Study the drawing (mm; zero at the part's minimum x, y, z) and answer. A direction names the side the tool comes from. Round coordinates to 2 decimals unless told otherwise and drop trailing zeros. Write each loop counter-clockwise with the first axis right and the second up, starting at its lowest first coordinate (ties: lowest second). Pieces come first, ordered by that corner, then holes. Notation, with made-up numbers: M -27,45.25 L -13,45.25 A34 cw -13,79.25 Z; hole C 2,68 d7. An arc over 180 degrees is marked long. Put each result on its own line as item: value. Start each with the question number.
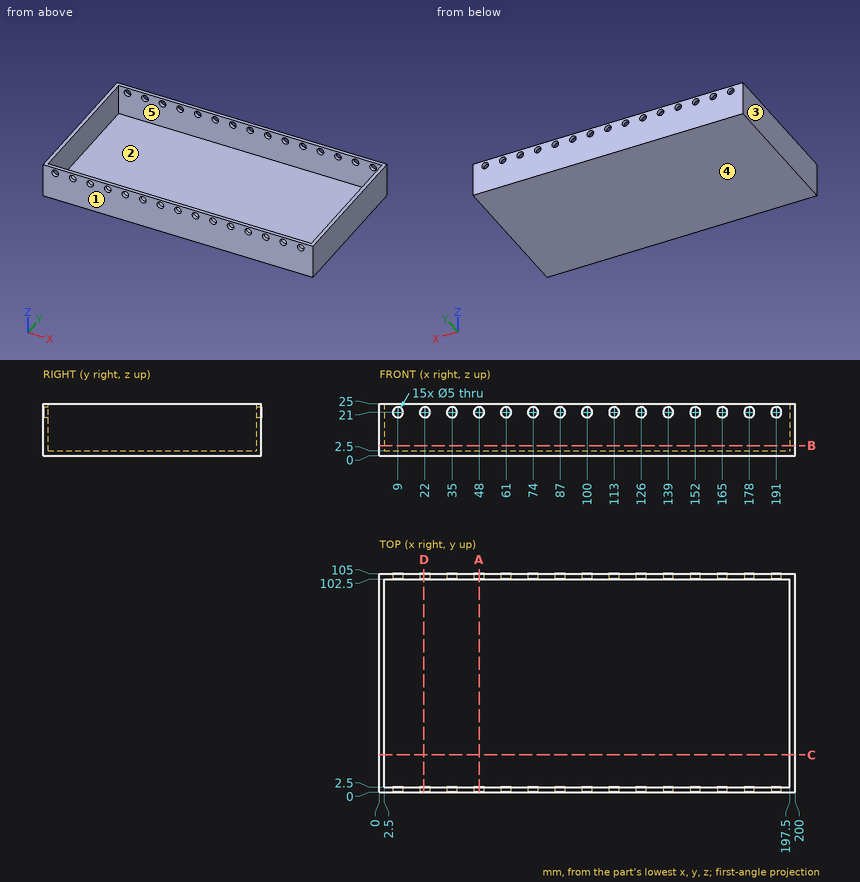
Item 1: Section A-A (x = 48) is taken. Give the vertices of the cut face in (y, z).
Item 2: Flat-ended cylindrical pins translate along their axes: pin 1 (3 mm diameter, centred on x = 176, y = 60, fed in from +Z); pin 2 (4.5 mm diameter, centred on x = 74, z = 21, fed in from +Y). Find the tip coordinate at first contact, or state that the pin passes through.
Item 3: Section B-B (z = 5) is taken. Give the vertices of the cut face in (x, y).
Item 4: Consider line 1 along X through (y, z) = (49.5, 13.25); line 2 along Z through (x, y) = (48, 0.95); line 3 along Y through (x, z) = (22, 17.25). Determine where each line is inside the solid, lowest interval first. Write a range as [from, to].
Item 5: Section C-C (y = 18) is taken. Give the vertices of the cut face in (x, z).
Item 6: Determine the mould class of the marked faces 1, 2 and 3 for opening direction Y: released by +Y, released by -Y, zero draft, split by the parting line, or undercut.
Item 7: Which of the six approach directions +Z, -Z, +X, -X, +Y, -Y give full straight-line access (tool end or side, diameter ignored) to the marked faces 4 and 5?
Item 8: Section D-D (x = 21.5) is taken. Give the vertices of the cut face in (y, z), and give its area (3 significant figures).
Output values:
1. outline: M 0,0 L 105,0 L 105,18.5 L 102.5,18.5 L 102.5,2.5 L 2.5,2.5 L 2.5,18.5 L 0,18.5 Z; M 0,23.5 L 2.5,23.5 L 2.5,25 L 0,25 Z; M 102.5,23.5 L 105,23.5 L 105,25 L 102.5,25 Z
2. pin 1: stops at z = 2.5
2. pin 2: passes through
3. outline: M 0,0 L 200,0 L 200,105 L 0,105 Z; hole M 2.5,2.5 L 197.5,2.5 L 197.5,102.5 L 2.5,102.5 Z
4. line 1: x = [0, 2.5], [197.5, 200]
4. line 2: z = [0, 18.5], [23.5, 25]
4. line 3: y = [0, 2.5], [102.5, 105]
5. outline: M 0,0 L 200,0 L 200,25 L 197.5,25 L 197.5,2.5 L 2.5,2.5 L 2.5,25 L 0,25 Z
6. face 1: released by -Y
6. face 2: undercut
6. face 3: zero draft
7. face 4: -Z, +X, -X, +Y, -Y
7. face 5: +Z
8. outline: M 0,0 L 105,0 L 105,18.55 L 102.5,18.55 L 102.5,2.5 L 2.5,2.5 L 2.5,18.55 L 0,18.55 Z; M 0,23.45 L 2.5,23.45 L 2.5,25 L 0,25 Z; M 102.5,23.45 L 105,23.45 L 105,25 L 102.5,25 Z
8. area: 351 mm^2
